from build123d import *

# Parameters (mm, degrees)
PAD_DEPTH       = 20
PAD001_DEPTH    = 20
SKETCH002_R     = 1.6
POCKET_DEPTH    = 262.582051
SKETCH003_W     = 9
SKETCH003_H     = 9
POCKET001_DEPTH = 1.5
CHAMFER_SIZE    = 5
FILLET_R        = 1
FILLET001_R     = 3
SKETCH004_R     = 5
SKETCH004_R_2   = 1.25
PAD002_DEPTH    = 4
SKETCH005_R     = 1.25
POCKET002_DEPTH = 46.001
CHAMFER001_SIZE = 2.5


with BuildPart() as part:
    # Sketch → Pad (new body)
    with BuildSketch(Plane.XY):
        Polygon((-41.5, -20.25), (-41.5, 20.25), (41.5, 20.25), (41.5, -20.25), (38.5, -20.25), (38.5, 17.25), (-38.5, 17.25), (-38.5, -20.25), align=None)
    extrude(amount=PAD_DEPTH)

    # Sketch001 (on Face9 of Pad) → Pad001 (join)
    with BuildSketch(Plane(origin=(0, 0, 0), x_dir=(1, 0, 0), z_dir=(0, 0, -1))):
        Polygon((-58.5, 20.25), (-58.5, 17.25), (-41.5, 17.25), (-41.5, 20.25), (-44, 20.25), (-45.75, 21.75), (-51.25, 21.75), (-53, 20.25), align=None)
    pad001 = extrude(amount=-PAD001_DEPTH)

    # Sketch002 (on Face2 of Pad001) → Pocket (cut, through all)
    with BuildSketch(Plane.XZ.offset(21.75)):
        with Locations((-48.5, 10)):
            Circle(SKETCH002_R)
    pocket = extrude(amount=-POCKET_DEPTH, mode=Mode.SUBTRACT)

    # Sketch003 (on Face5 of Pocket) → Pocket001 (cut)
    with BuildSketch(Plane.XZ.offset(21.75)):
        with Locations((-48.5, 10)):
            Rectangle(SKETCH003_W, SKETCH003_H)
    pocket001 = extrude(amount=-POCKET001_DEPTH, mode=Mode.SUBTRACT)

    # Mirrored: Pad001, Pocket, Pocket001 across Sketch001 V_Axis
    add(pad001.mirror(Plane(origin=(0, 0, 0), x_dir=(0, 0, -1), z_dir=(1, 0, 0))))
    add(pocket.mirror(Plane(origin=(0, 0, 0), x_dir=(0, 0, -1), z_dir=(1, 0, 0))), mode=Mode.SUBTRACT)
    add(pocket001.mirror(Plane(origin=(0, 0, 0), x_dir=(0, 0, -1), z_dir=(1, 0, 0))), mode=Mode.SUBTRACT)

    # Chamfer
    chamfer_edges = [part.edges().sort_by_distance(p)[0] for p in [
        (41.5, 20.25, 10),
        (38.5, 17.25, 10),
        (-41.5, 20.25, 10),
        (-38.5, 17.25, 10),
    ]]
    chamfer(chamfer_edges, length=CHAMFER_SIZE)

    # Fillet
    fillet_edges = [part.edges().sort_by_distance(p)[0] for p in [
        (38.5, -20.25, 10),
        (-38.5, -20.25, 10),
        (-41.5, -17.25, 10),
        (41.5, -17.25, 10),
    ]]
    fillet(fillet_edges, radius=FILLET_R)

    # Fillet001
    fillet001_edges = [part.edges().sort_by_distance(p)[0] for p in [
        (58.5, -18.75, 0),
        (58.5, -18.75, 20),
        (-58.5, -18.75, 0),
        (-58.5, -18.75, 20),
    ]]
    fillet(fillet001_edges, radius=FILLET001_R)

    # Sketch004 (on Face10 of Fillet001) → Pad002 (join)
    with BuildSketch(Plane(origin=(0, 20.25, 0), x_dir=(-1, 0, 0), z_dir=(0, 1, 0))):
        with Locations((-24.5, 10)):
            Circle(SKETCH004_R)
        with Locations((-24.5, 10)):
            Circle(SKETCH004_R_2, mode=Mode.SUBTRACT)
        with Locations((24.5, 10)):
            Circle(SKETCH004_R)
        with Locations((24.5, 10)):
            Circle(SKETCH004_R_2, mode=Mode.SUBTRACT)
    extrude(amount=PAD002_DEPTH)

    # Sketch005 (on Face47 of Pad002) → Pocket002 (cut, through all)
    with BuildSketch(Plane(origin=(0, 24.25, 0), x_dir=(-1, 0, 0), z_dir=(0, 1, 0))):
        with Locations((24.5, 10)):
            Circle(SKETCH005_R)
        with Locations((-24.5, 10)):
            Circle(SKETCH005_R)
    extrude(amount=-POCKET002_DEPTH, mode=Mode.SUBTRACT)

    # Chamfer001
    chamfer001_edges = [part.edges().sort_by_distance(p)[0] for p in [
        (29.5, 24.25, 10),
        (-19.5, 24.25, 10),
    ]]
    chamfer(chamfer001_edges, length=CHAMFER001_SIZE)


solid = part.part
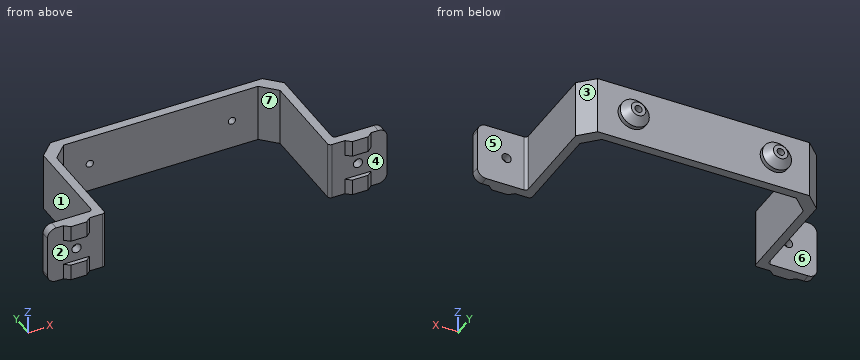
Could you check a few things on this model? Use its own coordinates, in mm. Face numbers are marked on the shaded views. A direction names the side the tool comes from. Coordinates: 2 decimals unless noted, no trailing zeros. Write each loop counter-clockwise with the first axis right and the second up, starting at its lowest first coordinate (ties: lowest second). Pieces come first, ordered by that corner, then holes. Notation, with made-up numbers: M 51,67.25 L 91,67.25 A29 ccw 91,93.25 Z; hole C 73,-6 d2. An arc over 180 degrees is marked long. One line per question, with ' | ' between items.
1) For the marked faces 4, 5, 6 and 7, which set-ups out of +Z, -Z, +X, -X, +Y, -Y let a thin tool reach every point of the face, with its end or its side?
Checks:
face 4: -Y | face 5: +Z, -Z, +X, +Y | face 6: +Z, -Z, -X, +Y | face 7: +Z, -Z, -Y
2) For pin 1 Ø2.5 at (x, z) = (-48.5, 10) entering from -Y; pin 2 Ø10 at (y, z) = (-3.5, 7.5) entering from -X; pin 3 Ø6 at (y, z) = (-11, 5.5) entering from +X; pin 4 Ø2 at (x, z) = (26, 16) entering from -Y, each with a flat end and sliding along its axis, tell me the tip position at first contact or that it passes through.
Checks:
pin 1: through | pin 2: x = -41.5 | pin 3: x = 41.5 | pin 4: y = 17.25
3) I need wall thicknesses on probe 1 along X at (y, z) = (12, 2.5); probe 2 along Y at (x, z) = (25.5, 16.5); probe 3 along X at (y, z) = (-19, 15.5). Which ranges of each line are inside material? Lowest first, please. Write a range as [from, to].
Checks:
probe 1: [-41.5, -38.5], [38.5, 41.5] | probe 2: [17.25, 20.25] | probe 3: [-58.5, -38.5], [38.5, 58.5]
4) Imagine slicing it at C-C, the plane z = 10. Give the number of separate pieces and of enclosed holes in the cut face, and give its area (3 significant figures).
Checks:
separate pieces: 5 | enclosed holes: 0 | area: 589 mm²
5) Imagine slicing it at D-D, the plane x = 24.5. Write out the boundary of the cut face in (y, z), and give its area (4 significant figures).
Checks:
outline: M 17.25,0 L 20.25,0 L 20.25,5 L 21.75,5 L 24.25,7.5 L 24.25,8.75 L 17.25,8.75 Z; M 17.25,11.25 L 24.25,11.25 L 24.25,12.5 L 21.75,15 L 20.25,15 L 20.25,20 L 17.25,20 Z | area: 76.25 mm²
6) Imagine slicing it at A-A, the plane x = -48.5. Write out the boundary of the cut face in (y, z), and give its area (3 significant figures).
Checks:
outline: M -21.75,0 L -17.25,0 L -17.25,8.4 L -20.25,8.4 L -20.25,5.5 L -21.75,5.5 Z; M -21.75,14.5 L -20.25,14.5 L -20.25,11.6 L -17.25,11.6 L -17.25,20 L -21.75,20 Z | area: 66.9 mm²
7) If we mould it in two halves opening along X, with no side actions, what happens to the marked faces 1, 2 and 3? For each: released by +X, released by -X, zero draft, split by the parting line, or undercut.
Checks:
face 1: released by -X | face 2: undercut | face 3: released by +X
8) Imagine slicing it at B-B, the plane y = -3. Write out the boundary of the cut face in (x, z), and give its area (3 significant figures).
Checks:
outline: M -41.5,0 L -38.5,0 L -38.5,20 L -41.5,20 Z; M 38.5,0 L 41.5,0 L 41.5,20 L 38.5,20 Z | area: 120 mm²
